Check sheet for the modelled part. Datum: model origin and axes. Units: mm. A direction names the side the tool comes from. Give positions to 0.01 mm unless a question says otherwise; leave off trailing zeros. Order: outer loops, then holes, each group sorted by start corner. A loop starts at its lowest first (then second) coordinate and runs counter-clockwise, first axis right, second up.
```python
from build123d import *

# Parameters (mm, degrees)
SKETCH_1_R      = 11
SKETCH_1_R_2    = 8
EXTRUDE_1_DEPTH = 10
EXTRUDE_START   = -5
SKETCH_2_R      = 8
SKETCH_2_R_2    = 5
EXTRUDE_2_DEPTH = 5


with BuildPart() as part:
    # Эскиз1 → Бобышка-Вытянуть1 (new body)
    with BuildSketch(Plane.XY):
        with BuildLine():
            Line((-27.5, 17.5), (27.5, 17.5))
            ThreePointArc((27.5, 17.5), (45, 0), (27.5, -17.5))
            Line((27.5, -17.5), (-27.5, -17.5))
            ThreePointArc((-27.5, -17.5), (-45, 0), (-27.5, 17.5))
        make_face()
        with Locations((-27.5, 0)):
            Circle(SKETCH_1_R, mode=Mode.SUBTRACT)
        with Locations((27.5, 0)):
            Circle(SKETCH_1_R_2, mode=Mode.SUBTRACT)
    extrude(amount=EXTRUDE_1_DEPTH)

    # Эскиз2 → Бобышка-Вытянуть2 (add)
    # profile 1 of 2: a face of its own
    with BuildSketch(Plane.XY.offset(10).offset(EXTRUDE_START)):
        with BuildLine():
            ThreePointArc((27.5, 17.5), (43.084968678, 7.959821059), (41.677549931, -10.258999852))
            Line((41.677549931, -10.258999852), (76.407572554, 37.736578368))
            ThreePointArc((76.407572554, 37.736578368), (64.46541326, 36.580250119), (64.806416341, 48.573414027))
            Line((64.806416341, 48.573414027), (27.5, 17.5))
        make_face()
    # profile 2 of 2: a face of its own
    with BuildSketch(Plane.XY.offset(10).offset(EXTRUDE_START)):
        with Locations((69.926406871, 42.426406871)):
            Circle(SKETCH_2_R)
        with Locations((69.926406871, 42.426406871)):
            Circle(SKETCH_2_R_2, mode=Mode.SUBTRACT)
    extrude(amount=EXTRUDE_2_DEPTH)


solid = part.part
```
(1) Cross-section at B-B on x = 31. Enter the section's corners in (y, z), then the cut area to 3 significant figures.
Response values:
outline: (-17.15, 0) - (-7.19, 0) - (-7.19, 10) - (-17.15, 10) - close; (7.19, 0) - (17.15, 0) - (17.15, 5) - (20.42, 5) - (20.42, 10) - (7.19, 10) - close
area: 215 mm2
(2) Gauge pin test, flat ends, axial feed: pin 1 Ø2 at (y, z) = (21.5, 2.5) entering from -X; pin 2 Ø5 at (x, y) = (55, 22.5) entering from -Z; pin 3 Ø6 at (x, z) = (57.5, 3.5) entering from -Y; pin 4 Ø6 at (x, y) = (37.5, -8) entering from -Z. Record the tip position at first contact, or that the pin passes through.
Response values:
pin 1: passes through
pin 2: stops at z = 5
pin 3: stops at y = 8.02
pin 4: stops at z = 0
(3) Cross-section at C-C on z = 3. Enter the section's corners in (x, y), then the cut area to 3 significant figures.
Response values:
outline: (-27.5, -17.5) - (27.5, -17.5) arc R17.5 ccw to (27.5, 17.5) - (-27.5, 17.5) arc R17.5 ccw to start; hole circle Ø22 at (-27.5, 0); hole circle Ø16 at (27.5, 0)
area: 2,310 mm2
(4) Set-up check for faces 1 (the face through (-17.339, -4.213, 4.93)), 2 (the face through (44.072, -5.622, 3.819)): record each of +Z, -Z, +X, -X, +Y, -Y from which the full face is reachable in a straight line by a thin tool's end or side.
Response values:
face 1: +Z, -Z
face 2: -Z, +X
(5) Release check for a two-part mould opening along Y. For faces 3 (the face through (54, 25, 5)), 4 (the face through (69.276, 47.384, 7.465)), 5 (the face through (19.508, 0.352, 4.93)), 6 (the face through (0, 17.5, 5)) record: released by +Y, released by -Y, zero draft, split by the parting line, or undercut.
Response values:
face 3: zero draft
face 4: undercut
face 5: undercut
face 6: released by +Y
(6) Material ranges on L1, parallel to Y at x = 27.5, z = 2.25; L2, parallel to X at y = 4.5, z = 1; L3, parallel to Y at x = 7, z = 6, recorded low to high.
Response values:
L1: y = -17.5 to -8, 8 to 17.5
L2: x = -44.41 to -37.54, -17.46 to 20.89, 34.11 to 44.41
L3: y = -17.5 to 17.5
(7) Cross-section at D-D on y = 0. Enter the section's corners in (x, z).
Response values:
outline: (-45, 0) - (-38.5, 0) - (-38.5, 10) - (-45, 10) - close; (-16.5, 0) - (19.5, 0) - (19.5, 10) - (-16.5, 10) - close; (35.5, 0) - (45, 0) - (45, 5) - (49.1, 5) - (49.1, 10) - (35.5, 10) - close
(8) Cross-section at A-A on y = 45.5. Enter the section's corners in (x, z).
Response values:
outline: (61.12, 5) - (65.98, 5) - (65.98, 10) - (61.12, 10) - close; (73.87, 5) - (77.31, 5) - (77.31, 10) - (73.87, 10) - close
